```python
from build123d import *

# Parameters (mm, degrees)
F1_DEPTH = 6.1
F3_DEPTH = 1.25


# Not quite as in the source:
# - a feature names something its author has since deleted; it is built from what else it names


with BuildPart() as f1:
    # F0 (on Top) → F1 (new body)
    with BuildSketch(Plane.XY):
        with BuildLine():
            ThreePointArc((12.5, 10.5), (11.9142135624, 11.9142135624), (10.5, 12.5))
            Line((10.5, 12.5), (4.5, 12.5))
            Line((4.5, 12.5), (4.5, 7.7))
            Line((4.5, 7.7), (-12.5, 7.7))
            Line((-12.5, 7.7), (-12.5, -10.5))
            ThreePointArc((-12.5, -10.5), (-11.9142135624, -11.9142135624), (-10.5, -12.5))
            Line((-10.5, -12.5), (10.5, -12.5))
            ThreePointArc((10.5, -12.5), (11.9142135624, -11.9142135624), (12.5, -10.5))
            Line((12.5, -10.5), (12.5, 10.5))
        make_face()
    extrude(amount=F1_DEPTH)

    # F2 (on face) → F3 (cut)
    with BuildSketch(Plane(origin=(0, 0, 0), x_dir=(1, 0, 0), z_dir=(0, 0, -1))):
        with BuildLine():
            ThreePointArc((10.5, -12.5), (11.9142135624, -11.9142135624), (12.5, -10.5))
            ThreePointArc((12.5, -10.5), (9.0857864376, -9.0857864376), (10.5, -12.5))
        make_face()
        with BuildLine():
            ThreePointArc((-8.5, 10.5), (-9.0857864376, 11.9142135624), (-10.5, 12.5))
            ThreePointArc((-10.5, 12.5), (-11.9142135624, 11.9142135624), (-12.5, 10.5))
            ThreePointArc((-12.5, 10.5), (-10.5, 8.5), (-8.5, 10.5))
        make_face()
    extrude(amount=-F3_DEPTH, mode=Mode.SUBTRACT)


solid = f1.part
```
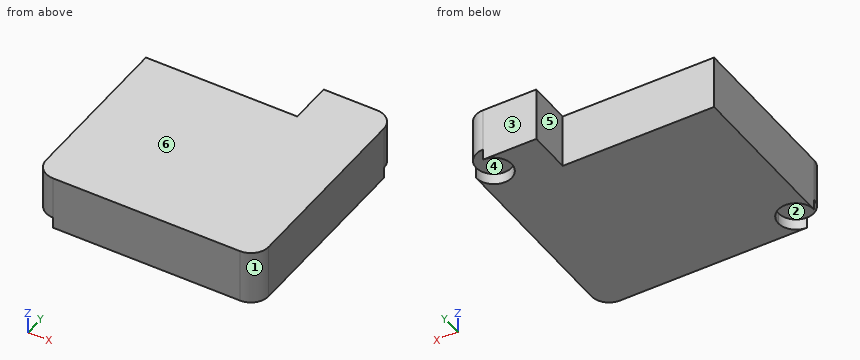
For this review, take the finished solid that the model builds, in its own axes (mm). Face numbers are marked on the shaded views. A direction names the side the tool comes from. Round coordinates to 2 decimals unless told otherwise and drop trailing zeros. Write each loop counter-clockwise with the first axis right and the second up, starting at its lowest first coordinate (ties: lowest second). Pieces come first, ordered by that corner, then holes. Notation, with made-up numbers: (22.5, -14) - (26.5, -14) arc R20 ccw to (26.5, 11) - close; hole circle Ø8 at (1.5, 62). An arc over 180 degrees is marked (long way). Answer as a JSON object with one key per item and string values.
1. Draft analysis for pull direction Y (two halves, no side actions). For the marked faces 1, 2, 3 and 4, state which applies: +Y half, -Y half, draft (parallel to the pull), parting line (faces both ways), or undercut.
Response values:
{"face 1": "-Y half", "face 2": "undercut", "face 3": "+Y half", "face 4": "undercut"}
2. We need section A-A on z = 5.75. Give the boundary of the cut face in (x, y).
Response values:
{"outline": "(-12.5, -10.5) arc R2 ccw to (-10.5, -12.5) - (10.5, -12.5) arc R2 ccw to (12.5, -10.5) - (12.5, 10.5) arc R2 ccw to (10.5, 12.5) - (4.5, 12.5) - (4.5, 7.7) - (-12.5, 7.7) - close"}
3. We need section B-B on y = -9.5. Give the boundary of the cut face in (x, z).
Response values:
{"outline": "(-12.5, 0) - (-12.23, 0) - (-12.23, 1.25) - (-8.77, 1.25) - (-8.77, 0) - (12.5, 0) - (12.5, 6.1) - (-12.5, 6.1) - close"}
4. To check wall thickness, follow line 1 along X through (y, z) = (9, 3); line 2 along Y through (x, z) = (0, 2.5); line 3 along Z through (x, y) = (-10, -10). State the ranges of each line that lie inside material, in increasing order.
Response values:
{"line 1": "x = 4.5 to 12.5", "line 2": "y = -12.5 to 7.7", "line 3": "z = 1.25 to 6.1"}
5. We need section D-D on x = 3.5. Give the boundary of the cut face in (y, z).
Response values:
{"outline": "(-12.5, 0) - (7.7, 0) - (7.7, 6.1) - (-12.5, 6.1) - close"}
6. For pin 1 Ø1.2 at (x, y) = (-9.5, -11) entering from -Z, flat-tipped, find the tip position at first contact; note if it passes through.
Response values:
{"pin 1": "stops at z = 1.25"}
7. Tool access review of the marked faces 5 and 6: name each direction out of +Z, -Z, +X, -X, +Y, -Y from which nothing blocks a thin tool from reaching the whole face with its end or side.
Response values:
{"face 5": "+Z, -Z, -X, +Y", "face 6": "+Z, +X, -X, +Y, -Y"}
8. We need section C-C on x = 9.5. Give the boundary of the cut face in (y, z), then the cut area to 3 significant figures.
Response values:
{"outline": "(-12.5, 0) - (8.77, 0) - (8.77, 1.25) - (12.23, 1.25) - (12.23, 0) - (12.5, 0) - (12.5, 6.1) - (-12.5, 6.1) - close", "area": "148 mm2"}
